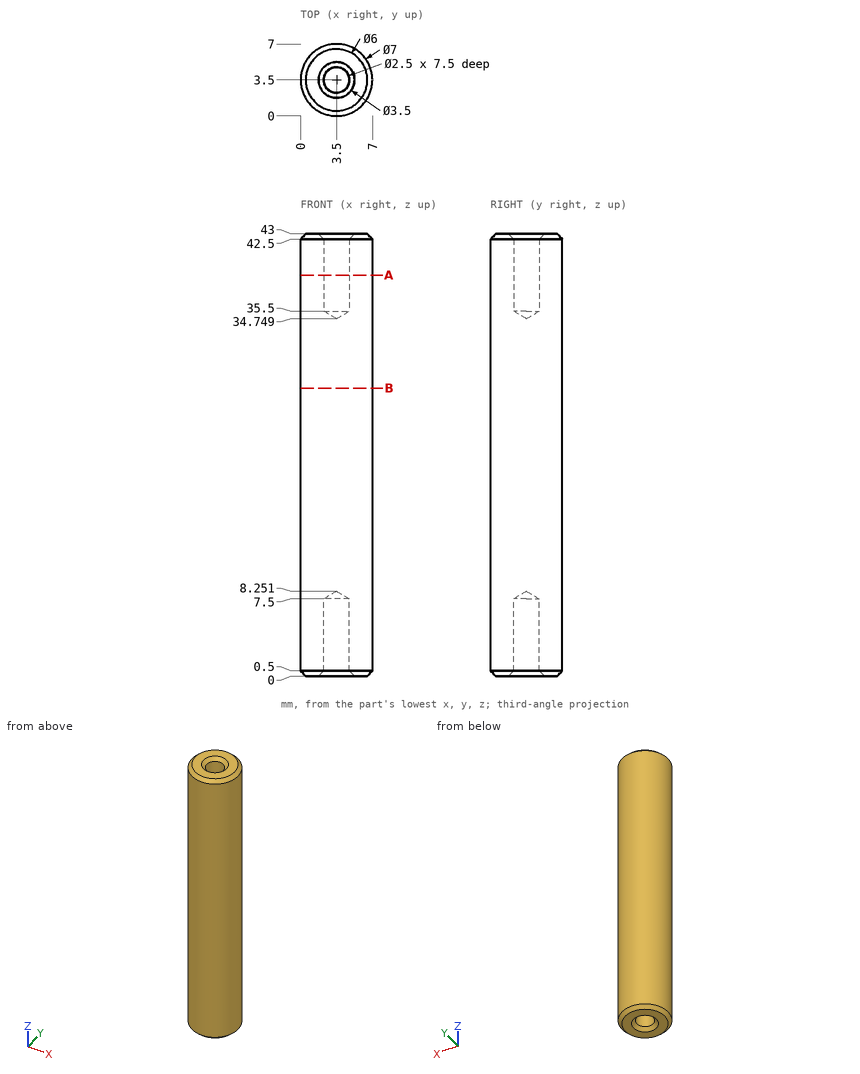
Input: dimensioned drawing with shaded views. Units: mm. Origin: part minimum x, y, z. Coordinates: 2 decimals unless noted, no trailing zeros. Order: outer loops, then holes, each group sorted by start corner. A loop starts at its lowest first (then second) coordinate and runs counter-clockwise, first axis right, second up. Notation, with made-up numbers: (-26, 44) - (-21, 44) arc R28 ccw to (-21, 77) - close; hole circle Ø8 at (15, -33). An arc over 180 degrees is marked (long way). One line per item, written item: value.
1) Contact query for flat-ended pins moving along their axis: pin 1 (2 mm diameter, centred on x = 0.5, z = 35.5, fed in from +Y); pin 2 (3 mm diameter, centred on x = 3.5, y = 3.5, fed in from +Z); pin 3 (1.5 mm diameter, centred on x = 1, z = 15.5, fed in from +Y); pin 4 (4 mm diameter, centred on x = 4, y = 4, fed in from +Z). Output: stop coordinate, or through.
Computed values:
pin 1: stops at y = 6.37
pin 2: stops at z = 42.75
pin 3: stops at y = 6.53
pin 4: stops at z = 43
2) Cut plane B-B on z = 28. Output: boundary loops of the cut face in (x, y).
Computed values:
outline: circle Ø7 at (3.5, 3.5)
3) Cut plane A-A on z = 39. Output: boundary loops of the cut face in (x, y).
Computed values:
outline: circle Ø7 at (3.5, 3.5); hole circle Ø2.5 at (3.5, 3.5)
4) Ray query, line 1 (Y direction, x = 3.5, z = 38.75); line 2 (X direction, y = 4.5, z = 4.5); line 3 (Z direction, x = 3, y = 4.75). Return the intervals inside material, ascending. Write a range as [from, to].
Computed values:
line 1: y = [0, 2.25], [4.75, 7]
line 2: x = [0.15, 2.75], [4.25, 6.85]
line 3: z = [0.4, 42.6]
